Geometry check sheet. Reference: drawing and pictorial views, mm from the part's lowest x, y, z. Give positions to 0.01 mm unless a question says otherwise; leave off trailing zeros. Order: outer loops, then holes, each group sorted by start corner. A loop starts at its lowest first (then second) coordinate and runs counter-clockwise, first axis right, second up. Notation, with made-up numbers: (-0.5, -33) - (38.5, -33) arc R33 ccw to (38.5, -3) - close; hole circle Ø10 at (-11, 24.5). An arc over 180 degrees is marked (long way). Answer in a Markdown table with one row per item.
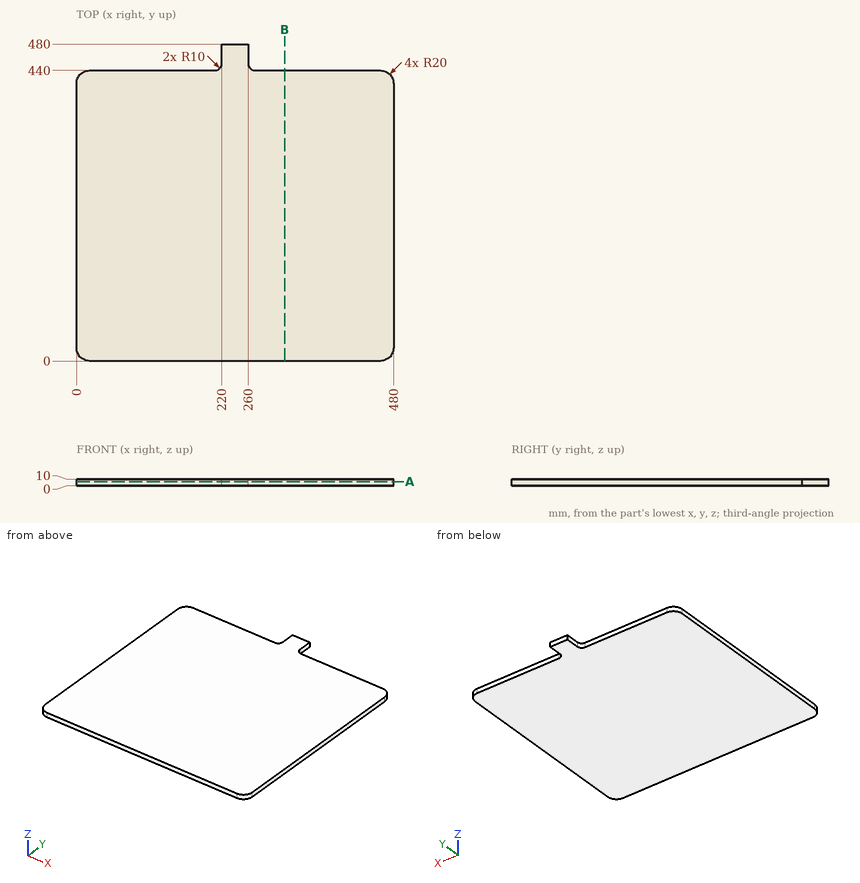
(1) Cross-section at B-B, the plane x = 315. Record the cut outline in (y, z).
Geometry says:
| item | result |
|---|---|
| outline | (0, 0) - (440, 0) - (440, 10) - (0, 10) - close |
(2) Thickness scan on L1, parallel to Y at x = 172, z = 7.25; L2, parallel to X at y = 452, z = 1.5; L3, parallel to X at y = 436.5, z = 5. Record the ranges inside material, lowest first.
Geometry says:
| item | result |
|---|---|
| L1 | 0 to 440 |
| L2 | 220 to 260 |
| L3 | 8.7 to 471.3 |
(3) Gauge pin test, flat ends, axial feed: P1, Ø2, axis at x = 165, y = 271.5, coming from the -Z side; P2, Ø5, axis at y = 468.5, z = 5, coming from the +X side; P3, Ø3, axis at x = 148.5, z = 7.5, coming from the +Y side. Record the tip position at first contact, or that the pin passes through.
Geometry says:
| item | result |
|---|---|
| P1 | z = 0 |
| P2 | x = 260 |
| P3 | y = 440 |
(4) Cross-section at A-A, the plane z = 6. Record the cut outline in (x, y), then the cut area to 4 significant figures.
Geometry says:
| item | result |
|---|---|
| outline | (0, 20) arc R20 ccw to (20, 0) - (460, 0) arc R20 ccw to (480, 20) - (480, 420) arc R20 ccw to (460, 440) - (270, 440) arc R10 cw to (260, 450) - (260, 480) - (220, 480) - (220, 450) arc R10 cw to (210, 440) - (20, 440) arc R20 ccw to (0, 420) - close |
| area | 212,500 mm² |
